from build123d import *

# Parameters (mm, degrees)
F0_R     = 6
F0_R_2   = 2
F0_W     = 42.228937149
F0_H     = 40
F0_R_3   = 3
F0_W_2   = 52
F0_H_2   = 26
F1_DEPTH = 5


# Not quite as in the source:
# - the program builds the solid bodies; features that only make, move or delete a surface that nothing else refers to are left out


with BuildPart() as f1:
    # F0 (on Front) → F1 (new body)
    with BuildSketch(Plane.XZ):
        with BuildLine():
            Line((114.488999566, 5.1368772984), (153.7277594005, 5.1368772984))
            ThreePointArc((153.7277594005, 5.1368772984), (206.6891166454, 35.9273670532), (230.521004176, 92.3631780006))
            Line((230.521004176, 92.3631780006), (37.6957547904, 92.3631780006))
            ThreePointArc((37.6957547904, 92.3631780006), (61.527642321, 35.9273670532), (114.488999566, 5.1368772984))
        make_face()
        with BuildLine():
            add(Edge.make_bspline(
                [(59.4798011976, 64.6672644662), (63.1085559726, 55.6081011891), (73.7513924788, 39.0135130084), (88.0385711789, 27.8172641993), (99.4798011976, 24.6672644662)],
                knots=[0, 0, 0, 0, 0.4955592973, 1, 1, 1, 1], degree=3))
            Line((59.4798011976, 64.6672644662), (99.4798011976, 64.6672644662))
            Line((99.4798011976, 64.6672644662), (99.4798011976, 24.6672644662))
        make_face(mode=Mode.SUBTRACT)
        with Locations((79.4798011976, 75.4959482996)):
            Circle(F0_R, mode=Mode.SUBTRACT)
        with Locations((68.8243359327, 77.2860795259)):
            Circle(F0_R_2, mode=Mode.SUBTRACT)
        with Locations((68.4796720743, 87.2811824083)):
            Circle(F0_R_2, mode=Mode.SUBTRACT)
        with Locations((78.4747824073, 87.6258462667)):
            Circle(F0_R_2, mode=Mode.SUBTRACT)
        with Locations((136.1386179924, 44.6672644662)):
            Rectangle(F0_W, F0_H, mode=Mode.SUBTRACT)
        with BuildLine():
            Line((169.434517622, 64.6672644662), (209.434517622, 64.6672644662))
            add(Edge.make_bspline(
                [(169.434517622, 24.6672644662), (179.2577588513, 27.1916796699), (196.3345264834, 41.3050241265), (205.696706141, 54.1838165912), (209.434517622, 64.6672644662)],
                knots=[0, 0, 0, 0, 0.5114020852, 1, 1, 1, 1], degree=3))
            Line((169.434517622, 24.6672644662), (169.434517622, 64.6672644662))
        make_face(mode=Mode.SUBTRACT)
        with BuildLine():
            Line((37.6957547904, 92.3631780006), (230.521004176, 92.3631780006))
            ThreePointArc((230.521004176, 92.3631780006), (230.8000531475, 101.1758471342), (230.2752492915, 109.9773007924))
            Line((230.2752492915, 109.9773007924), (37.941509675, 109.9773007924))
            ThreePointArc((37.941509675, 109.9773007924), (37.4167058189, 101.1758471342), (37.6957547904, 92.3631780006))
        make_face()
        with Locations((68.4796720743, 95.552995801)):
            Circle(F0_R_2, mode=Mode.SUBTRACT)
        with Locations((68.259306113, 104.66844666)):
            Circle(F0_R_2, mode=Mode.SUBTRACT)
        with Locations((187.7316534519, 101.4121994376)):
            Circle(F0_R_3, mode=Mode.SUBTRACT)
        with BuildLine():
            Line((37.941509675, 109.9773007924), (230.2752492915, 109.9773007924))
            ThreePointArc((230.2752492915, 109.9773007924), (134.1083794832, 196.5278747198), (37.941509675, 109.9773007924))
        make_face()
        with Locations((101.7344622612, 140.218708396)):
            Rectangle(F0_W_2, F0_H_2, mode=Mode.SUBTRACT)
        with BuildLine():
            Line((168.7307208776, 116.4853125811), (168.7307208776, 153.218708396))
            add(Edge.make_bspline(
                [(168.7307208776, 153.218708396), (178.5376432275, 150.9342291161), (199.0201954085, 146.7686018938), (211.3988850452, 126.7827873103), (217.8624719381, 116.4853125811)],
                knots=[0, 0, 0, 0, 0.4802466092, 1, 1, 1, 1], degree=3))
            Line((217.8624719381, 116.4853125811), (168.7307208776, 116.4853125811))
        make_face(mode=Mode.SUBTRACT)
    extrude(amount=-F1_DEPTH)


solid = f1.part
The model under review builds one solid part; all positions refer to its coordinate system, in mm. A direction names the side the tool comes from. Coordinates: 2 decimals unless noted, no trailing zeros. Loops run counter-clockwise (first coordinate to the right, second up) from the corner with the lowest first, then second, coordinate; pieces in that order, holes last.
(1) Tool access review of faces 3 (the flat face through (133, 5, 102)), 4 (the flat face through (101, 2, 127.219)): name each direction out of +Z, -Z, +X, -X, +Y, -Y from which nothing blocks a thin tool from reaching the whole face with its end or side.
Determined:
face 3: +Z, -Z, +X, -X, +Y
face 4: +Y, -Y
(2) Consider section D-D, the plane z = 167.5. Give the boundary of the cut face in (x, y).
Determined:
outline: (65.03, 0) - (203.18, 0) - (203.18, 5) - (65.03, 5) - close
(3) Wall thickness on L1, parallel to Z at x = 89.5, y = 4.7; L2, parallel to X at y = 2.1, z = 76; L3, parallel to Z at x = 84.5, y = 0.8: over which ranges is each line inside the solid? List them lowest first.
Determined:
L1: z = 14.03 to 28.52, 64.67 to 127.22, 153.22 to 185.62
L2: x = 40.39 to 67.29, 70.36 to 73.5, 85.46 to 227.83
L3: z = 16.82 to 31.52, 64.67 to 72.21, 78.78 to 127.22, 153.22 to 182.83
(4) Consider section A-A, the plane x = 138. Give the boundary of the cut face in (y, z), plus the area to 3 significant figures.
Determined:
outline: (0, 5.14) - (5, 5.14) - (5, 24.67) - (0, 24.67) - close; (0, 64.67) - (5, 64.67) - (5, 196.45) - (0, 196.45) - close
area: 757 mm2
(5) Consider section B-B, the plane z = 32.5. Give the number of separate pieces and of enclosed holes in the cut face, plus the area to 3 significant figures.
Determined:
separate pieces: 4
enclosed holes: 0
area: 324 mm2
(6) Draft analysis for pull direction X (two halves, no side actions). For faces 1 (the flat face through (133, 0, 102)), 2 (the flat face through (101, 2, 153.219)), state which applies: +X half, -X half, draft (parallel to the pull), parting line (faces both ways), or undercut.
Determined:
face 1: draft
face 2: undercut
(7) Insertion check: P1, Ø3, axis at y = 2.5, z = 166, coming from the -X side; P2, Ø1.5, axis at x = 184, y = 3.5, coming from the +Z side; P3, Ø1.5, axis at x = 103, y = 2.5, coming from the +Z side. Each pin has a flat end and moves straight along its axis. Give the tip position at first contact, or say it passes through.
Determined:
P1: stops at x = 62.22
P2: stops at z = 183.11
P3: stops at z = 191.64
